Check sheet for the modelled part. Datum: model origin and axes. Units: mm. A direction names the side the tool comes from. Round coordinates to 2 decimals unless told otherwise and drop trailing zeros. Write each loop counter-clockwise with the first axis right and the second up, starting at its lowest first coordinate (ties: lowest second). Pieces come first, ordered by that corner, then holes. Notation, with made-up numbers: (-24.5, -11.5) -> (2.5, -11.5) arc R14 ccw to (2.5, 2.5) -> close; hole circle Ø11 at (59.5, -4.75). An arc over 180 degrees is marked (long way). One line per item, written item: value.
from build123d import *

# Parameters (mm, degrees)
BOSS_EXTRUDE2_DEPTH     = 15.5
CUT_EXTRUDE1_DEPTH      = 24.510635891
CUT_EXTRUDE1_DEPTH_BACK = 24.510635891
SKETCH5_W               = 25
SKETCH5_H               = 21
SKETCH6_R               = 7.5
BOSS_EXTRUDE3_DEPTH     = 4
SKETCH7_R               = 7.5
BOSS_EXTRUDE4_DEPTH     = 4
CUT_EXTRUDE2_DEPTH      = 36.68613176
CUT_EXTRUDE2_DEPTH_BACK = 36.68613176
SKETCH8_R               = 3
BOSS_EXTRUDE6_DEPTH     = 31
CUT_EXTRUDE3_DEPTH      = 49.054656382
CUT_EXTRUDE3_DEPTH_BACK = 49.054656382
SKETCH11_R              = 3


with BuildPart() as part:
    # Sketch1 → Boss-Extrude2 (new, symmetric)
    with BuildSketch(Plane.XY):
        with BuildLine():
            Line((-12.5, 0), (-12.5, 12.5))
            Line((-12.5, 12.5), (12.5, 12.5))
            Line((12.5, 12.5), (12.5, 0))
            ThreePointArc((12.5, 0), (0, -12.5), (-12.5, 0))
        make_face()
    extrude(amount=BOSS_EXTRUDE2_DEPTH, both=True)

    # Sketch5 → Cut-Extrude1 (cut, two sides: drawn at the far end of the back side and taken through both)
    with BuildSketch(Plane(origin=(0, 0, 0), x_dir=(1, 0, 0), z_dir=(0, 1, 0)).offset(-CUT_EXTRUDE1_DEPTH_BACK)):
        Rectangle(SKETCH5_W, SKETCH5_H)
    extrude(amount=CUT_EXTRUDE1_DEPTH + CUT_EXTRUDE1_DEPTH_BACK, mode=Mode.SUBTRACT)


with BuildPart() as cut_extrude1_piece_1:
    # of the separate pieces the step leaves, piece 1, a body of its own (cut_extrude1_pieces)
    add(part.part.solids().sort_by_distance((-12.5, 0, -15.5))[0])

    # Sketch6 → Boss-Extrude3 (add)
    with BuildSketch(Plane.XY.offset(-10.5)):
        Circle(SKETCH6_R)
    extrude(amount=BOSS_EXTRUDE3_DEPTH)


with BuildPart() as cut_extrude1_piece_2:
    # of the separate pieces the step leaves, piece 2, a body of its own (cut_extrude1_pieces)
    add(part.part.solids().sort_by_distance((-12.5, 0, 10.5))[0])

    # Sketch7 → Boss-Extrude4 (add)
    with BuildSketch(Plane(origin=(0, 0, 10.5), x_dir=(-1, 0, 0), z_dir=(0, 0, -1))):
        Circle(SKETCH7_R)
    extrude(amount=BOSS_EXTRUDE4_DEPTH)


with BuildPart() as cut_extrude2_tool:
    # Sketch8 → Cut-Extrude2 (new, two sides: drawn at the far end of the back side and taken through both)
    with BuildSketch(Plane(origin=(0, 0, -15.5), x_dir=(-1, 0, 0), z_dir=(0, 0, -1)).offset(-CUT_EXTRUDE2_DEPTH_BACK)):
        Circle(SKETCH8_R)
    extrude(amount=CUT_EXTRUDE2_DEPTH + CUT_EXTRUDE2_DEPTH_BACK)


with BuildPart() as cut_extrude1_piece_1_1:
    add(cut_extrude1_piece_1.part)

    # Cut-Extrude2: cut by cut_extrude2_tool
    add(cut_extrude2_tool.part, mode=Mode.SUBTRACT)


with BuildPart() as cut_extrude1_piece_2_1:
    add(cut_extrude1_piece_2.part)

    # Cut-Extrude2: cut by cut_extrude2_tool
    add(cut_extrude2_tool.part, mode=Mode.SUBTRACT)

    # Sketch9 → Boss-Extrude6 (add)
    with BuildSketch(Plane.XY.offset(15.5)):
        with BuildLine():
            Line((12.5, 12.5), (12.5, 25.5))
            ThreePointArc((12.5, 25.5), (0, 38), (-12.5, 25.5))
            Line((-12.5, 25.5), (-12.5, 12.5))
            Line((-12.5, 12.5), (12.5, 12.5))
        make_face()
    extrude(amount=-BOSS_EXTRUDE6_DEPTH)

    # Sketch11 → Cut-Extrude3 (cut, two sides: drawn at the far end of the back side and taken through both)
    with BuildSketch(Plane(origin=(12.5, 0, 0), x_dir=(0, 0, -1), z_dir=(1, 0, 0)).offset(-CUT_EXTRUDE3_DEPTH_BACK)):
        with Locations((0, 25.5)):
            Circle(SKETCH11_R)
    extrude(amount=CUT_EXTRUDE3_DEPTH + CUT_EXTRUDE3_DEPTH_BACK, mode=Mode.SUBTRACT)


with BuildPart() as cut_extrude1_piece_1_2:
    add(cut_extrude1_piece_1_1.part)

    # Combine1: union Cut-Extrude1 piece 2
    add(cut_extrude1_piece_2_1.part)


solid = cut_extrude1_piece_1_2.part
Item 1: Sectioned sample at D-D on x = 10. Enter the section's corners in (y, z).
Answer:
outline: (-7.5, -15.5) -> (33, -15.5) -> (33, 15.5) -> (-7.5, 15.5) -> (-7.5, 10.5) -> (12.5, 10.5) -> (12.5, -10.5) -> (-7.5, -10.5) -> close; hole circle Ø6 at (25.5, 0)
Item 2: Sectioned sample at A-A on x = 0. Enter the section's corners in (y, z).
Answer:
outline: (-12.5, -15.5) -> (-3, -15.5) -> (-3, -6.5) -> (-7.5, -6.5) -> (-7.5, -10.5) -> (-12.5, -10.5) -> close; (-12.5, 10.5) -> (-7.5, 10.5) -> (-7.5, 6.5) -> (-3, 6.5) -> (-3, 15.5) -> (-12.5, 15.5) -> close; (3, -15.5) -> (38, -15.5) -> (38, 15.5) -> (3, 15.5) -> (3, 6.5) -> (7.5, 6.5) -> (7.5, 10.5) -> (12.5, 10.5) -> (12.5, -10.5) -> (7.5, -10.5) -> (7.5, -6.5) -> (3, -6.5) -> close; hole circle Ø6 at (25.5, 0)
Item 3: Sectioned sample at C-C on z = 0. Enter the section's corners in (x, y).
Answer:
outline: (-12.5, 12.5) -> (12.5, 12.5) -> (12.5, 22.5) -> (-12.5, 22.5) -> close; (-12.13, 28.5) -> (12.13, 28.5) arc R12.5 ccw to start
Item 4: Thickness scan on line 1 (Y direction, x = 0.5, z = 0); line 2 (Z direction, x = -8, y = 10); line 3 (Y direction, x = 0, z = 13.5). Record the ranges inside material, lowest first.
Answer:
line 1: y = 12.5 to 22.5, 28.5 to 37.99
line 2: z = -15.5 to -10.5, 10.5 to 15.5
line 3: y = -12.5 to -3, 3 to 38
Item 5: Sectioned sample at B-B on y = 9. Enter the section's corners in (x, z).
Answer:
outline: (-12.5, -15.5) -> (12.5, -15.5) -> (12.5, -10.5) -> (-12.5, -10.5) -> close; (-12.5, 10.5) -> (12.5, 10.5) -> (12.5, 15.5) -> (-12.5, 15.5) -> close
Item 6: Mould release check, pull along X, two halves, no side actions. Record for faces 6 (the cylindrical face through (3, 0, 11)), 7 (the flat face through (0, 8, 10.5)), 8 (the cylindrical face through (3, 0, -11)), 9 (the cylindrical face through (7.493, 0.33, 8.528)): pulls with the +X half, pulls with the -X half, needs draft (parallel to the pull), parting line crosses it, or undercut.
Answer:
face 6: undercut
face 7: needs draft
face 8: undercut
face 9: parting line crosses it
Item 7: Depth check by flat-ended pin: P1, Ø8, axis at y = 25.5, z = 0, coming from the -X side; P2, Ø6, axis at x = -7.5, z = 7.5, coming from the +Y side; P3, Ø1, axis at y = -3, z = -5, coming from the +X side; P4, Ø1, axis at y = 29, z = -10, coming from the -X side. Enter the tip coordinate at first touch or a pass-through.
Answer:
P1: stops at x = -12.5
P2: stops at y = 37.16
P3: passes through
P4: stops at x = -12.13
Item 8: Tool access check on faces 1 (the flat face through (0, 12.5, 0)), 2 (the flat face through (0, 13, -15.5)), 3 (the flat face through (3.2, 0.1, -6.5)), 4 (the flat face through (0, 8, -10.5)), 5 (the cylindrical face through (0.275, -12.497, -12.965)). Record the directions out of +Z, -Z, +X, -X, +Y, -Y that give a thin tool (end or side, any length) a straight path to the whole face; none if there is none.
Answer:
face 1: +X, -X
face 2: -Z, +X, -X, +Y, -Y
face 3: +X, -X, -Y
face 4: none
face 5: +Z, -Z, -Y
